Source: CAD feature listing. Evaluate the final solid. Frame: model axes, mm. A direction names the side the tool comes from. Give positions to 0.01 mm unless a question says otherwise; leave off trailing zeros. Order: outer loops, then holes, each group sorted by start corner. A loop starts at its lowest first (then second) coordinate and runs counter-clockwise, first axis right, second up. Notation, with made-up numbers: (79.25, 89.5) - (99.25, 89.5) arc R23 cw to (99.25, 105.5) - close; hole circle Ø5 at (77, -5.75). An arc over 180 degrees is marked (long way). One line per item, written item: value. Start each with the question number.
from build123d import *

# Parameters (mm, degrees)
CROQUIS1_W              = 75
CROQUIS1_H              = 70
SALIENTE_EXTRUIR1_DEPTH = 2
CROQUIS2_W              = 75
CROQUIS2_H              = 70
CROQUIS2_W_2            = 72
CROQUIS2_H_2            = 67
SALIENTE_EXTRUIR2_DEPTH = 25
CROQUIS3_R              = 1.525
CORTAR_EXTRUIR1_DEPTH   = 10


with BuildPart() as part:
    # Croquis1 → Saliente-Extruir1 (new body)
    with BuildSketch(Plane(origin=(0, 0, 0), x_dir=(1, 0, 0), z_dir=(0, 1, 0))):
        Rectangle(CROQUIS1_W, CROQUIS1_H)
    extrude(amount=SALIENTE_EXTRUIR1_DEPTH)

    # Croquis2 → Saliente-Extruir2 (add)
    with BuildSketch(Plane(origin=(0, 2, 0), x_dir=(1, 0, 0), z_dir=(0, 1, 0))):
        Rectangle(CROQUIS2_W, CROQUIS2_H)
        Rectangle(CROQUIS2_W_2, CROQUIS2_H_2, mode=Mode.SUBTRACT)
    extrude(amount=SALIENTE_EXTRUIR2_DEPTH)

    # Croquis3 → Cortar-Extruir1 (cut)
    with BuildSketch(Plane(origin=(0, 2, 0), x_dir=(1, 0, 0), z_dir=(0, 1, 0))):
        with Locations(Location((-29.21, 27.305, 0), (0, 0, 270))):
            Circle(CROQUIS3_R)
        with Locations(Location((-29.21, -27.305, 0), (0, 0, 270))):
            Circle(CROQUIS3_R)
        with Locations(Location((29.21, 27.305, 0), (0, 0, 270))):
            Circle(CROQUIS3_R)
        with Locations(Location((29.21, -27.3049805, 0), (0, 0, 270))):
            Circle(CROQUIS3_R)
    extrude(amount=-CORTAR_EXTRUIR1_DEPTH, mode=Mode.SUBTRACT)


solid = part.part
1. Draft query along Z for faces 3 (the flat face through (-1, 13, -35)), 4 (the flat face through (-1, 13, 35)), 5 (the flat face through (-36, 14, 0)). Return one class per face: pulls with the +Z half, pulls with the -Z half, needs draft (parallel to the pull), parting line crosses it, or undercut.
2. Ray query, L1, parallel to X at y = 22.75, z = 0.5; L2, parallel to Z at x = 1.5, y = 20.25; L3, parallel to Y at x = -26, z = -31.5. Return the intervals inside material, ascending.
3. Section A-A on x = 29.21. Return the cut outline in (y, z).
4. Contact query for flat-ended pins moving along their axis: pin 1 Ø4 at (x, z) = (29.21, 27.3) entering from +Y; pin 2 Ø2.5 at (x, z) = (-29.21, 27.305) entering from -Y. Output: stop coordinate, or through.
5. Section C-C on y = 16.25. Return the cut outline in (x, z), then the cut area to 3 significant figures.
6. Section B-B on z = -23. Return the cut outline in (x, y).
7. Set-up query: faces 1 (the flat face through (37.5, 13, 0)), 2 (the flat face through (36, 14, 0)). Return all of +Z, -Z, +X, -X, +Y, -Y with unobstructed straight access to the full face (end or side cutting, diameter ignored); none if empty.
8. Section D-D on x = 16.5. Return the cut outline in (y, z), then the cut area to 3 significant figures.
Data:
1. face 3: pulls with the -Z half
1. face 4: pulls with the +Z half
1. face 5: undercut
2. L1: x = -37.5 to -36, 36 to 37.5
2. L2: z = -35 to -33.5, 33.5 to 35
2. L3: y = 0 to 2
3. outline: (0, -35) - (27, -35) - (27, -33.5) - (2, -33.5) - (2, -28.83) - (0, -28.83) - close; (0, -25.78) - (2, -25.78) - (2, 25.78) - (0, 25.78) - close; (0, 28.83) - (2, 28.83) - (2, 33.5) - (27, 33.5) - (27, 35) - (0, 35) - close
4. pin 1: stops at y = 2
4. pin 2: passes through
5. outline: (-37.5, -35) - (37.5, -35) - (37.5, 35) - (-37.5, 35) - close; hole (-36, -33.5) - (36, -33.5) - (36, 33.5) - (-36, 33.5) - close
5. area: 426 mm2
6. outline: (-37.5, 0) - (37.5, 0) - (37.5, 27) - (36, 27) - (36, 2) - (-36, 2) - (-36, 27) - (-37.5, 27) - close
7. face 1: +Z, -Z, +X, +Y, -Y
7. face 2: +Y
8. outline: (0, -35) - (27, -35) - (27, -33.5) - (2, -33.5) - (2, 33.5) - (27, 33.5) - (27, 35) - (0, 35) - close
8. area: 215 mm2
